Geometry: final body of the model. Coordinates: model frame, mm. Give positions to 0.01 mm unless a question says otherwise; leave off trailing zeros. Write each loop counter-clockwise with the first axis right and the second up, starting at its lowest first coordinate (ties: lowest second). Pieces come first, ordered by that corner, then holes. Notation, with made-up numbers: M 32.25,57 L 72.25,57 A30 cw 72.25,88 Z; hole C -39,31.25 d4. An arc over 180 degrees is marked long. Use a Markdown table: item, result. Add a question column.
(1) Cut plane C-C (y = -1.7). State how many separate pieces and enclosed holes the cut face has, plus the area to 3 significant figures.
(2) Cut plane A-A (z = 71). Output: boundary loops of the cut face in (x, y) (3 decimals), plus the area to 3 significant figures.
(3) Material intervals for L1, parallel to X at y = -2.1, z = 106; L2, parallel to Z at x = -188, y = -1.25; L3, parallel to Z at x = 141, y = -0.6, sorted ascending.
(4) Cut plane B-B (x = 186). Output: boundary loops of the cut face in (y, z), plus the area to 3 significant figures.
(5) Pin query (flat end, axial travel): pin 1 Ø1 at (y, z) = (-2, 10) entering from -X; pin 2 Ø1.2 at (x, y) = (-140.5, -1) entering from +Z; pin 3 Ø1.2 at (y, z) = (-1.5, 151.5) entering from -X; pin 4 Ø6.5 at (x, z) = (208.45, 93.65) entering from -Y. Return the tip coordinate at first contact, or that it passes through.
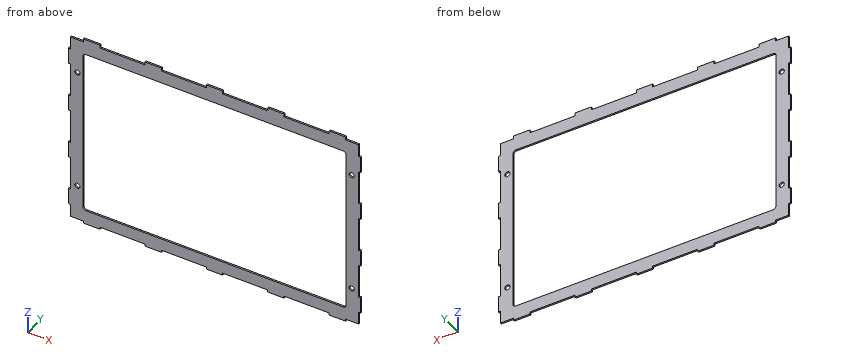
```python
from build123d import *

# Parameters (mm, degrees)
SKETCH1_W           = 438.5
SKETCH1_H           = 297.3
BASE_FLANGE1_DEPTH  = 2.5
SKETCH6_W           = 3
SKETCH6_H           = 25
BOSS_EXTRUDE1_DEPTH = 2.5
SKETCH8_W           = 25
SKETCH8_H           = 4.5
BOSS_EXTRUDE2_DEPTH = 2.5
SKETCH9_W           = 25
SKETCH9_H           = 3
BOSS_EXTRUDE3_DEPTH = 2.5
SKETCH10_W          = 0.35
SKETCH10_H          = 19.65
SKETCH10_W_2        = 20
SKETCH10_H_2        = 0.35
SKETCH10_H_3        = 52.4334
SKETCH10_H_4        = 20
SKETCH10_W_3        = 19.65
SKETCH10_W_4        = 68.375
SKETCH10_W_5        = 0.125
SKETCH10_H_5        = 52.4333
CUT_EXTRUDE1_DEPTH  = 10
SKETCH11_R          = 4
CUT_EXTRUDE2_DEPTH  = 3.05


# Sheet-metal steps are written as plain solids
with BuildPart() as part:
    # Sketch1 → Base-Flange1 (new body)
    with BuildSketch(Plane(origin=(0, 0, 0), x_dir=(1, 0, 0), z_dir=(0, 1, 0))):
        Rectangle(SKETCH1_W, SKETCH1_H)
        with BuildLine():
            Line((-195.2, 129.6), (195.2, 129.6))
            ThreePointArc((195.2, 129.6), (198.735533906, 128.135533906), (200.2, 124.6))
            Line((200.2, 124.6), (200.2, -123.65))
            ThreePointArc((200.2, -123.65), (198.735533906, -127.185533906), (195.2, -128.65))
            Line((195.2, -128.65), (-195.2, -128.65))
            ThreePointArc((-195.2, -128.65), (-198.735533906, -127.185533906), (-200.2, -123.65))
            Line((-200.2, -123.65), (-200.2, 124.6))
            ThreePointArc((-200.2, 124.6), (-198.735533906, 128.135533906), (-195.2, 129.6))
        make_face(mode=Mode.SUBTRACT)
    extrude(amount=-BASE_FLANGE1_DEPTH)

    # Sketch6 → Boss-Extrude1 (add)
    with BuildSketch(Plane(origin=(0, 0, 0), x_dir=(1, 0, 0), z_dir=(0, 1, 0))):
        with Locations((220.75, -116.15)):
            Rectangle(SKETCH6_W, SKETCH6_H)
        with Locations((220.75, -38.7166)):
            Rectangle(SKETCH6_W, SKETCH6_H)
        with Locations((220.75, 38.7167)):
            Rectangle(SKETCH6_W, SKETCH6_H)
        with Locations((220.75, 116.15)):
            Rectangle(SKETCH6_W, SKETCH6_H)
    boss_extrude1 = extrude(amount=-BOSS_EXTRUDE1_DEPTH)

    # Mirror1: Boss-Extrude1 across plane
    add(boss_extrude1.mirror(Plane(origin=(0, 0, 0), x_dir=(0, 0, 1), z_dir=(1, 0, 0))))

    # Sketch8 → Boss-Extrude2 (add)
    with BuildSketch(Plane(origin=(0, 0, 0), x_dir=(1, 0, 0), z_dir=(0, 1, 0))):
        with Locations((-186.75, -150.9)):
            Rectangle(SKETCH8_W, SKETCH8_H)
        with Locations((93.375, -150.9)):
            Rectangle(SKETCH8_W, SKETCH8_H)
        with Locations((-93.375, -150.9)):
            Rectangle(SKETCH8_W, SKETCH8_H)
        with Locations((0, -150.9)):
            Rectangle(SKETCH8_W, SKETCH8_H)
        with Locations((186.75, -150.9)):
            Rectangle(SKETCH8_W, SKETCH8_H)
    extrude(amount=-BOSS_EXTRUDE2_DEPTH)

    # Sketch9 → Boss-Extrude3 (add)
    with BuildSketch(Plane(origin=(0, 0, 0), x_dir=(1, 0, 0), z_dir=(0, 1, 0))):
        with Locations((-186.75, 150.15)):
            Rectangle(SKETCH9_W, SKETCH9_H)
        with Locations((-93.375, 150.15)):
            Rectangle(SKETCH9_W, SKETCH9_H)
        with Locations((0, 150.15)):
            Rectangle(SKETCH9_W, SKETCH9_H)
        with Locations((93.375, 150.15)):
            Rectangle(SKETCH9_W, SKETCH9_H)
        with Locations((186.75, 150.15)):
            Rectangle(SKETCH9_W, SKETCH9_H)
    extrude(amount=-BOSS_EXTRUDE3_DEPTH)

    # Sketch10 → Cut-Extrude1 (cut)
    with BuildSketch(Plane(origin=(0, 0, 0), x_dir=(1, 0, 0), z_dir=(0, 1, 0))):
        with Locations((219.075, 138.475)):
            Rectangle(SKETCH10_W, SKETCH10_H)
        with Locations((209.25, 148.475)):
            Rectangle(SKETCH10_W_2, SKETCH10_H_2)
        with Locations((-219.075, -77.4333)):
            Rectangle(SKETCH10_W, SKETCH10_H_3)
        with Locations((-219.075, -138.65)):
            Rectangle(SKETCH10_W, SKETCH10_H_4)
        with Locations((-209.075, -148.475)):
            Rectangle(SKETCH10_W_3, SKETCH10_H_2)
        with Locations((-140.0625, -148.475)):
            Rectangle(SKETCH10_W_4, SKETCH10_H_2)
        with Locations((-46.6875, -148.475)):
            Rectangle(SKETCH10_W_4, SKETCH10_H_2)
        with Locations((46.6875, -148.475)):
            Rectangle(SKETCH10_W_4, SKETCH10_H_2)
        with Locations((140.0625, -148.475)):
            Rectangle(SKETCH10_W_4, SKETCH10_H_2)
        with Locations((209.25, -148.475)):
            Rectangle(SKETCH10_W_2, SKETCH10_H_2)
        with Locations((219.075, -138.475)):
            Rectangle(SKETCH10_W, SKETCH10_H)
        with Locations((219.1875, -77.4333)):
            Rectangle(SKETCH10_W_5, SKETCH10_H_3)
        with Locations((219.075, 5e-05)):
            Rectangle(SKETCH10_W, SKETCH10_H_5)
        with Locations((219.075, 77.43335)):
            Rectangle(SKETCH10_W, SKETCH10_H_5)
        with Locations((140.0625, 148.475)):
            Rectangle(SKETCH10_W_4, SKETCH10_H_2)
        with Locations((46.6875, 148.475)):
            Rectangle(SKETCH10_W_4, SKETCH10_H_2)
        with Locations((-46.6875, 148.475)):
            Rectangle(SKETCH10_W_4, SKETCH10_H_2)
        with Locations((-209.25, 148.475)):
            Rectangle(SKETCH10_W_2, SKETCH10_H_2)
        with Locations((-140.0625, 148.475)):
            Rectangle(SKETCH10_W_4, SKETCH10_H_2)
        with Locations((-219.075, 138.475)):
            Rectangle(SKETCH10_W, SKETCH10_H)
        with Locations((-219.075, 77.43335)):
            Rectangle(SKETCH10_W, SKETCH10_H_5)
        with Locations((-219.075, 5e-05)):
            Rectangle(SKETCH10_W, SKETCH10_H_5)
    extrude(amount=-CUT_EXTRUDE1_DEPTH, mode=Mode.SUBTRACT)

    # Sketch11 → Cut-Extrude2 (cut)
    with BuildSketch(Plane(origin=(0, 0, 0), x_dir=(1, 0, 0), z_dir=(0, 1, 0))):
        with Locations(Location((-208.44992, 93.649, 0), (0, 0, 270))):
            Circle(SKETCH11_R)
        with Locations(Location((208.44992, 93.649, 0), (0, 0, 270))):
            Circle(SKETCH11_R)
        with Locations(Location((208.44992, -93.649, 0), (0, 0, 270))):
            Circle(SKETCH11_R)
        with Locations(Location((-208.44992, -93.649, 0), (0, 0, 270))):
            Circle(SKETCH11_R)
    extrude(amount=-CUT_EXTRUDE2_DEPTH, mode=Mode.SUBTRACT)


solid = part.part
```
Answer list:
| question | item | result |
|---|---|---|
| 1 | separate pieces | 1 |
| 1 | enclosed holes | 5 |
| 1 | area | 28,000 mm² |
| 2 | outline | M -218.9,-2.5 L -200.2,-2.5 L -200.2,0 L -218.9,0 Z; M 200.2,-2.5 L 219.125,-2.5 L 219.125,0 L 200.2,0 Z |
| 2 | area | 94.1 mm² |
| 3 | L1 | -222.25 to -200.2, 200.2 to 222.25 |
| 3 | L2 | -151.65 to -129.6, 128.65 to 153.15 |
| 3 | L3 | -148.3 to -129.6, 128.65 to 148.3 |
| 4 | outline | M -2.5,-151.65 L 0,-151.65 L 0,-129.6 L -2.5,-129.6 Z; M -2.5,128.65 L 0,128.65 L 0,153.15 L -2.5,153.15 Z |
| 4 | area | 116 mm² |
| 5 | pin 1 | x = -218.9 |
| 5 | pin 2 | z = 148.3 |
| 5 | pin 3 | x = -199.25 |
| 5 | pin 4 | through |
